Geometry: final body of the model. Coordinates: model frame, mm. Face numbers are marked on the shaded views. A direction names the side the tool comes from. Give positions to 0.01 mm unless a question says otherwise; leave off trailing zeros. Order: outer loops, then holes, each group sorted by start corner. A loop starts at its lowest first (then second) coordinate and runs counter-clockwise, first axis right, second up. Notation, with made-up numbers: (-28.75, 59) - (29.25, 59) arc R18 ccw to (29.25, 85) - close; hole circle Ø3 at (-2.5, 38). An arc over 180 degrees is marked (long way). One line per question, with ' | ' between items. Start each with the question number.
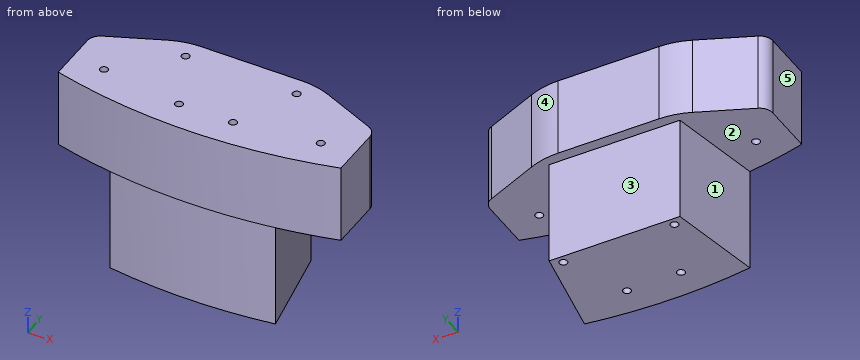
from build123d import *

# Parameters (mm, degrees)
F1_DEPTH = 30
F2_R     = 1.5
F3_DEPTH = 30.001
F4_R     = 28.5239911769
F5_R     = 5
F7_R     = 1.5
F8_DEPTH = 40


with BuildPart() as f1:
    # F0 (on Top) → F1 (new body)
    with BuildSketch(Plane.XY):
        with BuildLine():
            Line((-53.4347956585, -180.2462832153), (-53.4347956585, -203.0879676715))
            ThreePointArc((-53.4347956585, -203.0879676715), (0, -210), (53.4347956585, -203.0879676715))
            Line((53.4347956585, -203.0879676715), (53.4347956585, -180.2462832153))
            Line((53.4347956585, -180.2462832153), (25, -168))
            Line((25, -168), (0, -168))
            Line((0, -168), (-25, -168))
            Line((-25, -168), (-53.4347956585, -180.2462832153))
        make_face()
    extrude(amount=F1_DEPTH)

    # F2 (on face) → F3 (cut, through all)
    with BuildSketch(Plane.XY.offset(30)):
        with Locations((-61.4929363222, -189.1117421473)):
            Circle(F2_R)
        with Locations((-116.9707156809, -160.8515617902)):
            Circle(F2_R)
        with Locations((-161.0003432552, -116.8309564779)):
            Circle(F2_R)
        with Locations((-189.2718923255, -61.3589697679)):
            Circle(F2_R)
        with Locations((-199.0179466895, 0.1344137845)):
            Circle(F2_R)
        with Locations((61.4958267934, -189.0991398316)):
            Circle(F2_R)
        with Locations((116.9678135034, -160.8275907612)):
            Circle(F2_R)
        with Locations((160.9884188157, -116.7979631869)):
            Circle(F2_R)
        with Locations((189.2485991728, -61.3201838282)):
            Circle(F2_R)
        with Locations((198.9820512211, 0.175195735)):
            Circle(F2_R)
        with Locations((-20.9999999994, -175.0021517963)):
            Circle(F2_R)
        with Locations((-40.9903269079, -194.4499816389)):
            Circle(F2_R)
        with Locations((-10.2028351662, -198.7382755147)):
            Circle(F2_R)
        with Locations((20.9999997802, -174.9978481734)):
            Circle(F2_R)
        with Locations((10.2076995225, -198.7361841041)):
            Circle(F2_R)
        with Locations((40.9943117987, -194.4415809015)):
            Circle(F2_R)
    extrude(amount=-F3_DEPTH, mode=Mode.SUBTRACT)

    # F4
    f4_edges = [f1.edges().sort_by_distance(p)[0] for p in [
        (25, -168, 15),
        (-25, -168, 15),
    ]]
    fillet(f4_edges, radius=F4_R)

    # F5
    f5_edges = [f1.edges().sort_by_distance(p)[0] for p in [
        (53.434796, -180.246283, 15),
        (-53.434796, -180.246283, 15),
    ]]
    fillet(f5_edges, radius=F5_R)

    # F7 (on face) → F8 (join)
    with BuildSketch(Plane(origin=(0, 0, 0), x_dir=(1, 0, 0), z_dir=(0, 0, -1))):
        with BuildLine():
            ThreePointArc((31.2604393052, 207.6602632533), (0, 210), (-31.2604393052, 207.6602632533))
            Line((-31.2604393052, 207.6602632533), (-24.7243543685, 172.0646172762))
            Line((-24.7243543685, 172.0646172762), (0, 172.0646172762))
            Line((0, 172.0646172762), (24.7243543685, 172.0646172762))
            Line((24.7243543685, 172.0646172762), (31.2604393052, 207.6602632533))
        make_face()
        with Locations((-20.9999999994, 175.0021517963)):
            Circle(F7_R, mode=Mode.SUBTRACT)
        with Locations((20.9999997802, 174.9978481734)):
            Circle(F7_R, mode=Mode.SUBTRACT)
        with Locations((-10.2028351662, 198.7382755147)):
            Circle(F7_R, mode=Mode.SUBTRACT)
        with Locations((10.2076995225, 198.7361841041)):
            Circle(F7_R, mode=Mode.SUBTRACT)
    extrude(amount=F8_DEPTH)


solid = f1.part
(1) Cut plane D-D, the plane x = -37. Return the cut outline in (y, z), plus the area to 3 significant figures.
(2) Access query for the marked faces 1, 2 and 3. Directions: +Z, -Z, +X, -X, +Y, -Y. A direction counts if a zero-diameter tool reaches every point of the face in a straight line with its end or side. Return the directions, or none.
(3) Pull-direction query (Y, two-part tool) for the marked faces 4 and 5; classes: +Y half, -Y half, draft (parallel to the pull), parting line (faces both ways), or undercut.
(4) Material intervals for line 1 along X through (y, z) = (-195.5, 15); line 2 along Y through (x, z) = (11, -11); line 3 along Y through (x, z) = (1, -17.5), sorted ascending. Write a range as from..to.
(5) Cut plane B-B, the plane z = -25. Return the cut outline in (x, y), plus the area to 3 significant figures.
(6) Contact query for flat-ended pins moving along their axis: P1, Ø20, axis at x = 1.5, z = -18.5, coming from the +Y side; P2, Ø1, axis at x = 19, z = 17.5, coming from the -Y side; P3, Ø1, axis at x = -22.5, z = 19, coming from the +Y side. Output: stop coordinate, or through.
(7) Cut plane A-A, the plane x = -21. Return the cut outline in (y, z), plus the area to 3 significant figures.
(8) Cut plane C-C, the plane y = -191. Return the cut outline in (x, z).
Results are:
1) outline: (-206.71, 0) - (-173.17, 0) - (-173.17, 30) - (-206.71, 30) - close | area: 1,010 mm2
2) face 1: -Z, -X, +Y | face 2: -Z, +Y | face 3: -Z, +X, -X, +Y
3) face 4: +Y half | face 5: draft
4) line 1: -53.43..-42.06, -39.92..39.93, 42.06..53.43 | line 2: -209.71..-200.01, -197.46..-172.06 | line 3: -210..-172.06
5) outline: (-31.26, -207.66) arc R210 ccw to (31.26, -207.66) - (24.72, -172.06) - (-24.72, -172.06) - close; hole circle Ø3 at (-21, -175); hole circle Ø3 at (-10.2, -198.74); hole circle Ø3 at (10.21, -198.74); hole circle Ø3 at (21, -175) | area: 2,060 mm2
6) P1: y = -172.06 | P2: y = -209.18 | P3: y = -168.15
7) outline: (-208.95, -40) - (-176.5, -40) - (-176.5, 30) - (-208.95, 30) - close; (-173.5, -40) - (-172.06, -40) - (-172.06, 0) - (-168.06, 0) - (-168.06, 30) - (-173.5, 30) - close | area: 2,490 mm2
8) outline: (-53.43, 0) - (-28.2, 0) - (-28.2, -40) - (28.2, -40) - (28.2, 0) - (53.43, 0) - (53.43, 30) - (-53.43, 30) - close
